The listing builds one solid part. Answer for the finished solid, in the listing's coordinates (mm). A direction names the side the tool comes from. Coordinates: 2 decimals unless noted, no trailing zeros. Order: outer loops, then holes, each group sorted by start corner. A loop starts at its lowest first (then second) coordinate and runs counter-clockwise, first axis right, second up. Notation, with made-up numbers: (-36.5, 28) - (3.5, 28) arc R6 cw to (3.5, 32) - close; hole circle Ø4 at (-17.5, -30.75). An arc over 180 degrees is marked (long way). Use a Markdown table: item, result. Add a question column.
Item 1: Find the intervals of material crossed by line 1 along Z through (x, y) = (-7.8, 1.05); line 2 along Z through (x, y) = (-7.8, 0.6); line 3 along Z through (x, y) = (7.8, 0.4), in increasing order.
Item 2: The mould has two halves that part along Z. Classify faces 4 (the cylindrical face through (-8.75, 0.54, 4.98)), 5 (the flat face through (2.763, 2, 0)), 6 (the flat face through (-0.1, 0.5, 7)), 7 (the flat face through (4, 2, -1.878)): released by +Z, released by -Z, zero draft, split by the parting line, or undercut.
Item 3: For faces 1 (the flat face through (-9.5, 0.5, 1)), 2 (the flat face through (-6.054, 2, 1)), 3 (the flat face through (-3, 2.5, -1)), determine the directions among +Z, -Z, +X, -X, +Y, -Y from which every point of the face is accessible in a straight line to the end or side of a thin tool.
Item 4: The part is cut by section C-C, the plane y = 3.25. Give the vertices of the cut face in (x, z).
Item 5: Flat-ended cylindrical pins translate along their axes: P1, Ø0.8, axis at x = -2.5, y = 1.5, coming from the -Z side; P2, Ø1.4, axis at x = -7.8, z = -3, coming from the +Y side; P3, Ø1.2, axis at x = -3, y = 2, coming from the +Z side. Find the tip coordinate at first contact, or state that the pin passes through.
Item 6: The part is cut by section A-A, the plane z = -1.5. Give the vertices of the cut face in (x, y).
Item 7: The part is cut by section B-B, the plane x = 8. State how many separate pieces and enclosed holes the cut face has, then the cut area to 3 significant figures.
Item 8: The part is cut by section D-D, the plane z = -5.54. Give the vertices of the cut face in (x, y), then the cut area to 3 significant figures.
from build123d import *

# Parameters (mm, degrees)
SKETCH_1_W          = 19
SKETCH_1_H          = 14
EXTRUDE_1_DEPTH     = 1
SKETCH_2_R          = 0.75
SKETCH_2_R_2        = 0.602396592
CUT_EXTRUDE_1_DEPTH = 2
SKETCH_4_R          = 1.862700745
EXTRUDE_2_DEPTH     = 3
SKETCH_3_R          = 0.602396592
EXTRUDE_3_DEPTH     = 0.1
SKETCH_5_W          = 2.390465956
SKETCH_5_H          = 3.756446502
SKETCH_5_W_2        = 2.111060845
SKETCH_5_H_2        = 3.290771316
SKETCH_5_W_3        = 1.986880794
SKETCH_5_H_3        = 3.042411217
SKETCH_5_W_4        = 3.694356478
SKETCH_5_H_4        = 1.769565707
SKETCH_5_W_5        = 1.676430671
SKETCH_5_H_5        = 2.763006106
EXTRUDE_4_DEPTH     = 1.5


with BuildPart() as part:
    # Эскиз1 → Бобышка-Вытянуть1 (new body)
    with BuildSketch(Plane(origin=(0, 0, 0), x_dir=(1, 0, 0), z_dir=(0, 1, 0))):
        Rectangle(SKETCH_1_W, SKETCH_1_H)
    extrude(amount=EXTRUDE_1_DEPTH)

    # Эскиз2 → Вырез-Вытянуть1 (cut, through all)
    with BuildSketch(Plane(origin=(0, 1, 0), x_dir=(1, 0, 0), z_dir=(0, 1, 0))):
        with Locations((-9.5, -5)):
            Circle(SKETCH_2_R)
        with Locations((-9.5, 3)):
            Circle(SKETCH_2_R)
        with Locations((9.5, 3)):
            Circle(SKETCH_2_R)
        with Locations((9.5, -5)):
            Circle(SKETCH_2_R)
        with Locations((9.5, 5.54)):
            Circle(SKETCH_2_R)
        with Locations((-7.8, 3)):
            Circle(SKETCH_2_R_2)
        with Locations((-7.8, -5)):
            Circle(SKETCH_2_R_2)
        with Locations((7.8, 3)):
            Circle(SKETCH_2_R_2)
        with Locations((7.8, -5)):
            Circle(SKETCH_2_R_2)
        with Locations((7.8, 5.54)):
            Circle(SKETCH_2_R_2)
    extrude(amount=-CUT_EXTRUDE_1_DEPTH, mode=Mode.SUBTRACT)

    # Эскиз4 → Бобышка-Вытянуть2 (add)
    with BuildSketch(Plane(origin=(0, 1, 0), x_dir=(1, 0, 0), z_dir=(0, 1, 0))):
        with Locations((-3.383906354, 4.734364394)):
            Circle(SKETCH_4_R)
        with Locations((1.616093646, 4.734364394)):
            Circle(SKETCH_4_R)
    extrude(amount=EXTRUDE_2_DEPTH)

    # Эскиз3 → Бобышка-Вытянуть3 (add)
    with BuildSketch(Plane(origin=(0, 1, 0), x_dir=(1, 0, 0), z_dir=(0, 1, 0))):
        with BuildLine():
            Line((-7.668118067, -3.821776661), (-9.5, -3.821776661))
            Line((-9.5, -3.821776661), (-9.5, -4.25))
            ThreePointArc((-9.5, -4.25), (-8.75, -5), (-9.5, -5.75))
            Line((-9.5, -5.75), (-9.5, -6.178223339))
            Line((-9.5, -6.178223339), (-7.668118067, -6.178223339))
            ThreePointArc((-7.668118067, -6.178223339), (-6.489894728, -5), (-7.668118067, -3.821776661))
        make_face()
        with Locations((-7.8, -5)):
            Circle(SKETCH_3_R, mode=Mode.SUBTRACT)
        with BuildLine():
            Line((-9.5, 2.25), (-9.5, 1.821776661))
            Line((-9.5, 1.821776661), (-7.668118067, 1.821776661))
            ThreePointArc((-7.668118067, 1.821776661), (-6.489894728, 3), (-7.668118067, 4.178223339))
            Line((-7.668118067, 4.178223339), (-9.5, 4.178223339))
            Line((-9.5, 4.178223339), (-9.5, 3.75))
            ThreePointArc((-9.5, 3.75), (-8.75, 3), (-9.5, 2.25))
        make_face()
        with Locations((-7.8, 3)):
            Circle(SKETCH_3_R, mode=Mode.SUBTRACT)
        with BuildLine():
            Line((7.668118067, -6.178223339), (9.5, -6.178223339))
            Line((9.5, -6.178223339), (9.5, -5.75))
            ThreePointArc((9.5, -5.75), (8.75, -5), (9.5, -4.25))
            Line((9.5, -4.25), (9.5, -3.821776661))
            Line((9.5, -3.821776661), (7.668118067, -3.821776661))
            ThreePointArc((7.668118067, -3.821776661), (6.489894728, -5), (7.668118067, -6.178223339))
        make_face()
        with Locations((7.8, -5)):
            Circle(SKETCH_3_R, mode=Mode.SUBTRACT)
        with BuildLine():
            Line((9.5, 6.29), (9.5, 6.718223339))
            Line((9.5, 6.718223339), (7.668118067, 6.718223339))
            ThreePointArc((7.668118067, 6.718223339), (6.489894728, 5.54), (7.668118067, 4.361776661))
            Line((7.668118067, 4.361776661), (9.5, 4.361776661))
            Line((9.5, 4.361776661), (9.5, 4.79))
            ThreePointArc((9.5, 4.79), (8.75, 5.54), (9.5, 6.29))
        make_face()
        with Locations((7.8, 5.54)):
            Circle(SKETCH_3_R, mode=Mode.SUBTRACT)
        with BuildLine():
            Line((7.668118067, 1.821776661), (9.5, 1.821776661))
            Line((9.5, 1.821776661), (9.5, 2.25))
            ThreePointArc((9.5, 2.25), (8.75, 3), (9.5, 3.75))
            Line((9.5, 3.75), (9.5, 4.178223339))
            Line((9.5, 4.178223339), (7.668118067, 4.178223339))
            ThreePointArc((7.668118067, 4.178223339), (6.489894728, 3), (7.668118067, 1.821776661))
        make_face()
        with Locations((7.8, 3)):
            Circle(SKETCH_3_R, mode=Mode.SUBTRACT)
    extrude(amount=EXTRUDE_3_DEPTH)

    # Эскиз5 → Бобышка-Вытянуть4 (add)
    with BuildSketch(Plane(origin=(0, 1, 0), x_dir=(1, 0, 0), z_dir=(0, 1, 0))):
        with Locations((-3.026888711, -2.297330919)):
            Rectangle(SKETCH_5_W, SKETCH_5_H)
        with Locations((3.818536528, 0.232837593)):
            Rectangle(SKETCH_5_W_2, SKETCH_5_H_2)
        with Locations((-7.047217819, -0.82269283)):
            Rectangle(SKETCH_5_W_3, SKETCH_5_H_3)
        with Locations((-2.747483599, 1.303890522)):
            Rectangle(SKETCH_5_W_4, SKETCH_5_H_4)
        with Locations((7.82334313, -0.962395385)):
            Rectangle(SKETCH_5_W_5, SKETCH_5_H_5)
    extrude(amount=EXTRUDE_4_DEPTH)


solid = part.part
Solution:
| question | item | result |
|---|---|---|
| 1 | line 1 | z = -4.18 to -3.6, -2.4 to -1.82, -0.7 to 2.34, 3.82 to 4.4, 5.6 to 6.18 |
| 1 | line 2 | z = -7 to -3.6, -2.4 to 4.4, 5.6 to 7 |
| 1 | line 3 | z = -7 to -6.14, -4.94 to -3.6, -2.4 to 4.4, 5.6 to 7 |
| 2 | face 4 | undercut |
| 2 | face 5 | zero draft |
| 2 | face 6 | released by +Z |
| 2 | face 7 | undercut |
| 3 | face 1 | +Z, -Z, -X, +Y, -Y |
| 3 | face 2 | +Z, -Z, +Y |
| 3 | face 3 | +Z, +X, -X, +Y |
| 4 | outline | circle Ø3.73 at (-3.38, -4.73); circle Ø3.73 at (1.62, -4.73) |
| 5 | P1 | stops at z = -6.53 |
| 5 | P2 | stops at y = 1.1 |
| 5 | P3 | stops at z = 4.18 |
| 6 | outline | (-9.5, 0) - (9.5, 0) - (9.5, 1) - (4.87, 1) - (4.87, 2.5) - (2.76, 2.5) - (2.76, 1) - (-0.9, 1) - (-0.9, 2.5) - (-4.59, 2.5) - (-4.59, 1) - (-9.5, 1) - close |
| 7 | separate pieces | 4 |
| 7 | enclosed holes | 0 |
| 7 | area | 15.1 mm2 |
| 8 | outline | (-9.5, 0) - (7.2, 0) - (7.2, 1.1) - (6.49, 1.1) - (6.49, 1) - (3.3, 1) - (3.3, 4) - (-0.06, 4) - (-0.06, 1) - (-1.7, 1) - (-1.7, 4) - (-5.06, 4) - (-5.06, 1) - (-9.5, 1) - close; (8.4, 0) - (8.75, 0) - (8.75, 1.1) - (8.4, 1.1) - close |
| 8 | area | 37.3 mm2 |
